```python
from build123d import *

# Parameters (mm, degrees)
BOSS_EXTRUDE1_DEPTH = 2.54
SKETCH2_R           = 9.525
CUT_EXTRUDE1_DEPTH  = 19.05
SKETCH3_W           = 236.278650797
SKETCH3_H           = 2.54
BOSS_EXTRUDE2_DEPTH = 7.62
CUT_EXTRUDE2_DEPTH  = 3.54
FILLET1_R           = 10.16


with BuildPart() as part:
    # Sketch1 → Boss-Extrude1 (new body)
    with BuildSketch(Plane.XY.offset(-12.457776114)):
        Polygon((-279.4, 85.357628122), (127, 85.357628122), (127, 21.857628122), (0, 21.857628122), (0, -12.141055663), (-279.4, -12.141055663), align=None)
        with BuildLine():
            Line((-233.58, 19.833203878), (-68.58, 19.833203878))
            ThreePointArc((-68.58, 19.833203878), (-66.675, 17.928203878), (-68.58, 16.023203878))
            Line((-68.58, 16.023203878), (-233.58, 16.023203878))
            ThreePointArc((-233.58, 16.023203878), (-235.485, 17.928203878), (-233.58, 19.833203878))
        make_face(mode=Mode.SUBTRACT)
    extrude(amount=-BOSS_EXTRUDE1_DEPTH)

    # Sketch2 → Cut-Extrude1 (cut)
    with BuildSketch(Plane.XY.offset(-12.457776114)):
        with Locations((18.627536258, 29.178203878)):
            Circle(SKETCH2_R)
    extrude(amount=-CUT_EXTRUDE1_DEPTH, mode=Mode.SUBTRACT)

    # Sketch3 → Boss-Extrude2 (add)
    with BuildSketch(Plane.XY.offset(-12.457776114)):
        with Locations((-118.139325399, 25.548203878)):
            Rectangle(SKETCH3_W, SKETCH3_H)
        with Locations((-118.139325399, 10.308203878)):
            Rectangle(SKETCH3_W, SKETCH3_H)
    extrude(amount=BOSS_EXTRUDE2_DEPTH)

    # Sketch4 → Cut-Extrude2 (cut, through all)
    with BuildSketch(Plane.XY.offset(-12.457776114)):
        Polygon((-279.4, -12.141055663), (0, -12.141055663), (0, 9.038203878), (-236.955667324, 9.038203878), (-236.955667324, 27.294063936), (-3.574037437, 27.294063936), (-3.574037437, 50.510436651), (38.627466089, 50.510436651), (38.627466089, 2.859516917), (133.335307594, 2.859516917), (133.335307594, 92.146273099), (38.627466089, 92.146273099), (38.627466089, 93.769303319), (-279.4, 93.769303319), align=None)
    extrude(amount=-CUT_EXTRUDE2_DEPTH, mode=Mode.SUBTRACT)

    # Fillet1
    fillet1_edges = [part.edges().sort_by_distance(p)[0] for p in [
        (0, 21.857628122, -13.727776114),
        (-3.574037437, 27.294063936, -13.727776114),
        (38.627466089, 21.857628122, -13.727776114),
        (-3.574037437, 50.510436651, -13.727776114),
        (38.627466089, 50.510436651, -13.727776114),
    ]]
    fillet(fillet1_edges, radius=FILLET1_R)


solid = part.part
```
Design review of the part built by this model. Coordinates are the model's own, in mm. A direction names the side the tool comes from. Round coordinates to 2 decimals unless told otherwise and drop trailing zeros. Order: outer loops, then holes, each group sorted by start corner. A loop starts at its lowest first (then second) coordinate and runs counter-clockwise, first axis right, second up. Notation, with made-up numbers: M 45.25,22.5 L 101.25,22.5 A15 cw 101.25,46.5 Z; hole C -14.5,39 d4. An arc over 180 degrees is marked long. Put each result on its own line as item: value.
Q1. To check wall thickness, follow line 1 (Y direction, x = -96.5, z = -12.5); line 2 (Y direction, x = -215, z = -9); line 3 (Z direction, x = -22, y = 27). State the ranges of each line that lie inside material, in increasing order.
Reported:
line 1: 9.04 to 16.02, 19.83 to 27.29
line 2: 9.04 to 11.58, 24.28 to 26.82
line 3: -15 to -12.46
Q2. Insertion check: pin 1 Ø3 at (y, z) = (37.5, -12) entering from -X; pin 2 Ø3 at (x, z) = (-146.5, -13) entering from +Y; pin 3 Ø2 at (x, z) = (27, -14) entering from -Y. Each pin has a flat end and moves straight along its axis. Give the tip position at first contact, or say it passes through.
Reported:
pin 1: x = -3.67
pin 2: y = 27.29
pin 3: y = 21.86
Q3. Consider section B-B (x = 18). State the section outline as (y, z) points, and give its area (3 significant figures).
Reported:
outline: M 38.68,-15 L 50.51,-15 L 50.51,-12.46 L 38.68,-12.46 Z
area: 30.0 mm²
Q4. Consider section A-A (x = -182). State the section outline as (y, z) points, and give its area (3 significant figures).
Reported:
outline: M 9.04,-15 L 16.02,-15 L 16.02,-12.46 L 11.58,-12.46 L 11.58,-4.84 L 9.04,-4.84 Z; M 19.83,-15 L 27.29,-15 L 27.29,-12.46 L 26.82,-12.46 L 26.82,-4.84 L 24.28,-4.84 L 24.28,-12.46 L 19.83,-12.46 Z
area: 75.4 mm²
Q5. Machinability: for faces 4 (the face through (-120, 24.278, -9)), 5 (the face through (-120, 26.818, -9)), 6 (the face through (2.897, 18.802, -13.746)), which of the approach directions +Z, -Z, +X, -X, +Y, -Y give a long, thin tool a straight path to every point of the face, cutting with its end or side? Answer none if there is none.
Reported:
face 4: +Z, +X, -X
face 5: +Z, +X, -X, +Y
face 6: +Z, -Z, +X, -Y
Q6. Draft analysis for pull direction Y (two halves, no side actions). For faces 1 (the face through (-68, 21, -12.458)), 2 (the face through (-120, 9.038, -10)), 3 (the face through (-97, 21, -14.998)), state which applies: released by +Y, released by -Y, zero draft, split by the parting line, or undercut.
Reported:
face 1: undercut
face 2: released by -Y
face 3: zero draft
